```python
from build123d import *

# Parameters (mm, degrees)
F0_W     = 75
F0_H     = 75
F0_R     = 2.5
F0_R_2   = 15
F1_DEPTH = 5
F2_SIZE  = 3


with BuildPart() as f1:
    # F0 (on Front) → F1 (new body)
    with BuildSketch(Plane.XZ):
        with Locations((37.5, 37.5)):
            Rectangle(F0_W, F0_H)
        with Locations((10, 10)):
            Circle(F0_R, mode=Mode.SUBTRACT)
        with Locations((65, 10)):
            Circle(F0_R, mode=Mode.SUBTRACT)
        with Locations((10, 65)):
            Circle(F0_R, mode=Mode.SUBTRACT)
        with Locations((37.5, 37.5)):
            Circle(F0_R_2, mode=Mode.SUBTRACT)
        with Locations((65, 65)):
            Circle(F0_R, mode=Mode.SUBTRACT)
    extrude(amount=F1_DEPTH)

    # F2
    f2_edges = [f1.edges().sort_by_distance(p)[0] for p in [
        (75, -5, 37.5),
        (37.5, -5, 0),
        (37.5, -5, 75),
        (0, -5, 37.5),
        (7.5, -5, 65),
        (7.5, -5, 10),
        (62.5, -5, 10),
        (62.5, -5, 65),
    ]]
    chamfer(f2_edges, length=F2_SIZE)


solid = f1.part
```
Can you work these out from the model? Positions are in its coordinate system, mm. Give positions to 0.01 mm unless a question says otherwise; leave off trailing zeros. Loops run counter-clockwise (first coordinate to the right, second up) from the corner with the lowest first, then second, coordinate; pieces in that order, holes last. Notation, with made-up numbers: M 66.25,9 L 93.25,9 A29 cw 93.25,34 Z; hole C -21,3 d7. An arc over 180 degrees is marked long. One line per question, with ' | ' between items. Start each with the question number.
Q1. If I drill on line 1 (Z direction, x = 9, y = -2.1); line 2 (X direction, y = -3.7, z = 63); line 3 (X direction, y = -3.8, z = 11), over which ranges is the centre line in solid material (lowest first)? Write a range as from..to.
Q2. For pin 1 Ø6.5 at (x, z) = (65, 10) entering from -Y; pin 2 Ø4.5 at (x, z) = (10, 65) entering from -Y, each with a flat end and sliding along its axis, tell me the tip position at first contact or that it passes through.
Q3. If we section it at C-C (x = 37.5): Please give me the cut outline in (y, z).
Q4. If we section it at B-B (z = 10): Please give me the cut outline in (x, y), plus the area to 3 significant figures.
Q5. If we section it at A-A (z = 37.5): Please give me the cut outline in (x, y), plus the area to 3 significant figures.
Q6. If we section it at D-D (y = -0.8): Please give me the cut outline in (x, z), plus the area to 3 significant figures.
Computed:
1) line 1: z = 0.1..7.6, 12.4..62.6, 67.4..74.9 | line 2: x = 1.7..6.31, 13.69..61.31, 68.69..73.3 | line 3: x = 1.8..5.82, 14.18..60.82, 69.18..73.2
2) pin 1: stops at y = -2.75 | pin 2: passes through
3) outline: M -5,3 L -2,0 L 0,0 L 0,22.5 L -5,22.5 Z; M -5,52.5 L 0,52.5 L 0,75 L -2,75 L -5,72 Z
4) outline: M 0,-2 L 3,-5 L 4.5,-5 L 7.5,-2 L 7.5,0 L 0,0 Z; M 12.5,-2 L 15.5,-5 L 59.5,-5 L 62.5,-2 L 62.5,0 L 12.5,0 Z; M 67.5,-2 L 70.5,-5 L 72,-5 L 75,-2 L 75,0 L 67.5,0 Z | area: 298 mm²
5) outline: M 0,-2 L 3,-5 L 22.5,-5 L 22.5,0 L 0,0 Z; M 52.5,-5 L 72,-5 L 75,-2 L 75,0 L 52.5,0 Z | area: 216 mm²
6) outline: M 0,0 L 75,0 L 75,75 L 0,75 Z; hole C 10,10 d5; hole C 10,65 d5; hole C 37.5,37.5 d30; hole C 65,10 d5; hole C 65,65 d5 | area: 4,840 mm²
